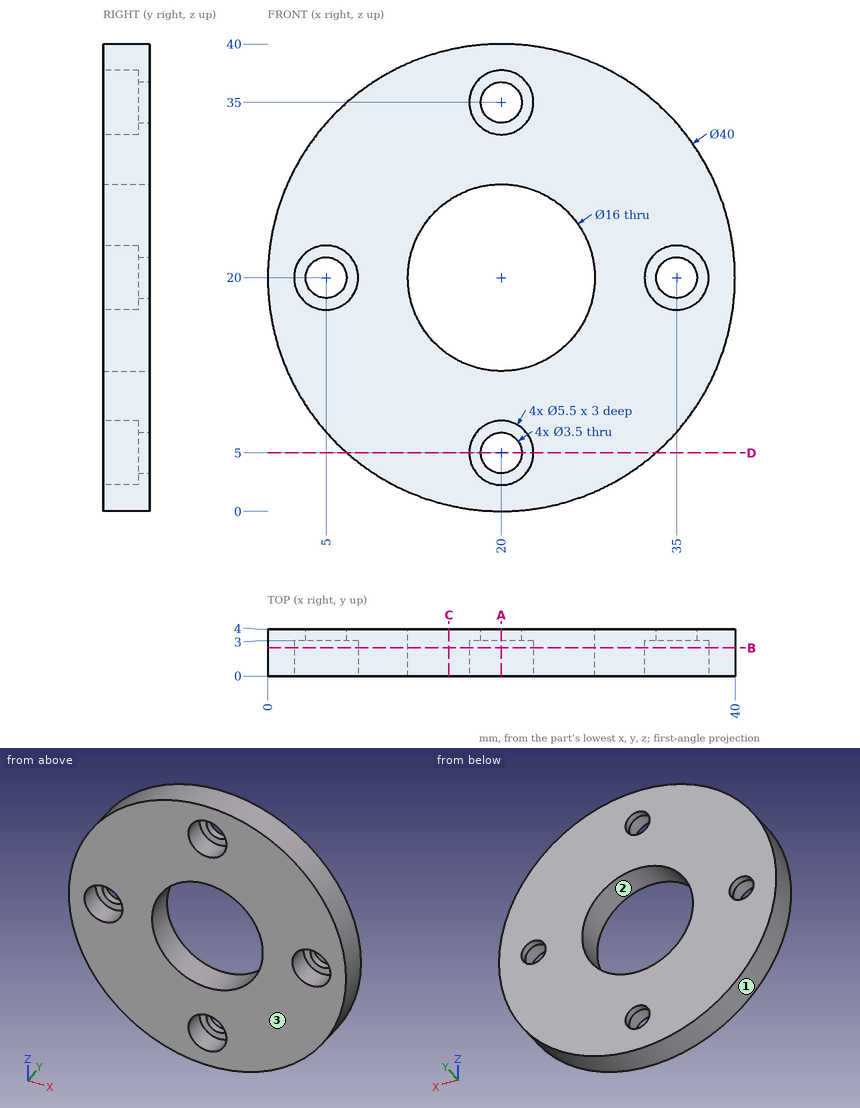
Check sheet for the drawn part. Datum: minimum x, y, z corner. Units: mm. Coordinates: 2 decimals unless noted, no trailing zeros. Loops run counter-clockwise (first coordinate to the right, second up) from the corner with the lowest first, then second, coordinate; pieces in that order, holes last. Notation, with made-up numbers: (-6, 79.5) -> (7, 79.5) arc R9 ccw to (7, 91.5) -> close; hole circle Ø10 at (-22.5, 43). An arc over 180 degrees is marked (long way). Write each question's results on one line, items separated by ' | '.
Item 1: Section check D-D, the plane z = 5. Enter the section's corners in (x, y).
Found:
outline: (6.77, 0) -> (17.25, 0) -> (17.25, 3) -> (18.25, 3) -> (18.25, 4) -> (6.77, 4) -> close; (21.75, 3) -> (22.75, 3) -> (22.75, 0) -> (33.23, 0) -> (33.23, 4) -> (21.75, 4) -> close
Item 2: Section check B-B, the plane y = 2.4. Enter the section's corners in (x, z), plus the area to 3 significant figures.
Found:
outline: circle Ø40 at (20, 20); hole circle Ø5.5 at (5, 20); hole circle Ø16 at (20, 20); hole circle Ø5.5 at (20, 5); hole circle Ø5.5 at (20, 35); hole circle Ø5.5 at (35, 20) | area: 961 mm2
Item 3: Material ranges on L1, parallel to Z at x = 20, y = 3.55; L2, parallel to Z at x = 20, y = 1.9; L3, parallel to Z at x = 32.5, y = 1.05, recorded low to high.
Found:
L1: z = 0 to 3.25, 6.75 to 12, 28 to 33.25, 36.75 to 40 | L2: z = 0 to 2.25, 7.75 to 12, 28 to 32.25, 37.75 to 40 | L3: z = 4.39 to 18.85, 21.15 to 35.61
Item 4: Section check A-A, the plane x = 20. Enter the section's corners in (y, z), plus the area to 3 significant figures.
Found:
outline: (0, 0) -> (4, 0) -> (4, 3.25) -> (3, 3.25) -> (3, 2.25) -> (0, 2.25) -> close; (0, 7.75) -> (3, 7.75) -> (3, 6.75) -> (4, 6.75) -> (4, 12) -> (0, 12) -> close; (0, 28) -> (4, 28) -> (4, 33.25) -> (3, 33.25) -> (3, 32.25) -> (0, 32.25) -> close; (0, 37.75) -> (3, 37.75) -> (3, 36.75) -> (4, 36.75) -> (4, 40) -> (0, 40) -> close | area: 56.0 mm2
Item 5: Gauge pin test, flat ends, axial feed: pin 1 (1.6 mm diameter, centred on x = 34.5, z = 19, fed in from -Y); pin 2 (1.5 mm diameter, centred on y = 3, z = 12.5, fed in from +X); pin 3 (1 mm diameter, centred on x = 28, y = 1.5, fed in from -Z). Record the tip position at first contact, or that the pin passes through.
Found:
pin 1: stops at y = 3 | pin 2: stops at x = 38.83 | pin 3: stops at z = 1.46
Item 6: Section check C-C, the plane x = 15.5. Enter the section's corners in (y, z).
Found:
outline: (0, 0.51) -> (4, 0.51) -> (4, 13.39) -> (0, 13.39) -> close; (0, 26.61) -> (4, 26.61) -> (4, 39.49) -> (0, 39.49) -> close
Item 7: Mould release check, pull along Z, two halves, no side actions. Record for the marked faces 1, 2 and 3: +Z half, -Z half, draft (parallel to the pull), parting line (faces both ways), or undercut.
Found:
face 1: parting line | face 2: undercut | face 3: draft
